Geometry: see drawing. Coordinates: mm, zero at the bounding-box minimum. Give positions to 0.01 mm unless a question says otherwise; leave off trailing zeros. Order: outer loops, then holes, each group sorted by start corner. A loop starts at its lowest first (then second) coordinate and runs counter-clockwise, first axis right, second up. Notation, with made-up numbers: (44.5, 25.5) -> (80.5, 25.5) arc R14 cw to (80.5, 52.5) -> close; hole circle Ø7 at (-28.5, -27). An arc over 180 degrees is marked (long way). One line per item, written item: value. Start each with the question number.
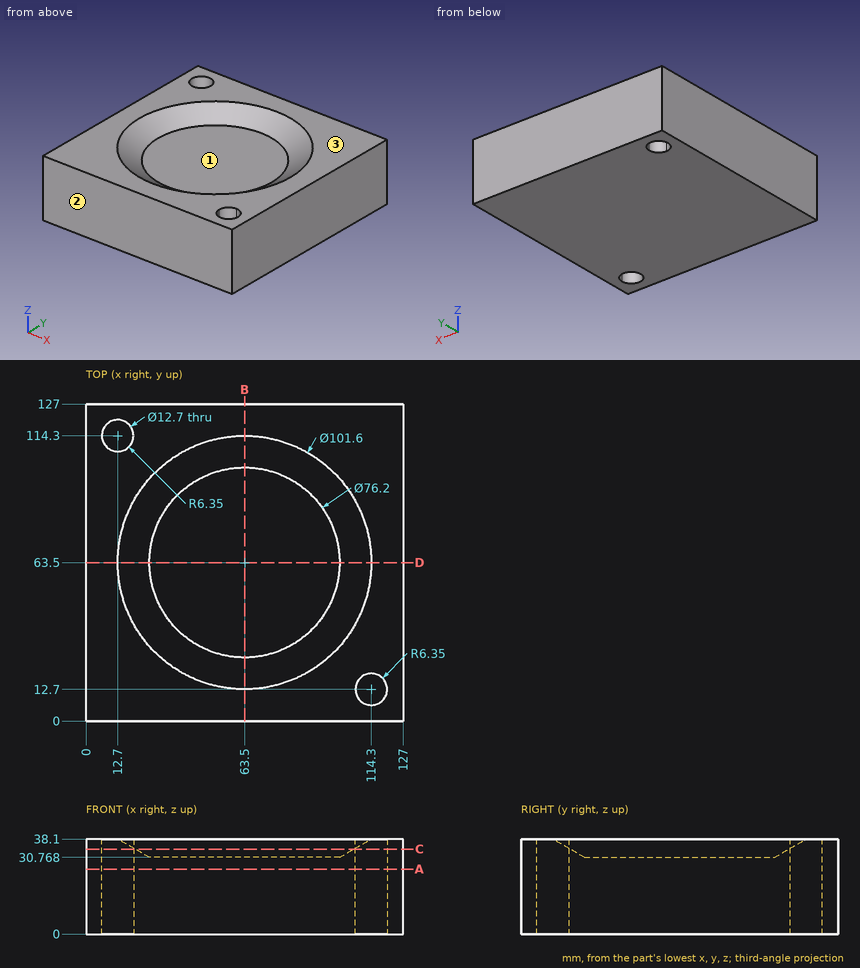
1. Cut plane B-B, the plane x = 63.5. Return loops of the section in (y, z), then the cut area to 3 significant figures.
2. Cut plane C-C, the plane z = 34. Return loops of the section in (x, y), then the cut area to 3 significant figures.
3. Pin query (flat end, axial travel): P1, Ø3, axis at x = 67.5, y = 35, coming from the +Z side; P2, Ø7.5, axis at x = 12.7, y = 114.3, coming from the -Z side. Return the tip coordinate at first contact, or that it passes through.
4. Cut plane A-A, the plane z = 26. Return loops of the section in (x, y), then the cut area to 3 significant figures.
5. Material intervals for L1, parallel to X at y = 114.3, z = 12; L2, parallel to Z at x = 43.5, y = 83; L3, parallel to Y at x = 12, z = 21, sorted ascending. Write a range as [from, to].
6. Draft query along Y for the marked faces 1, 2 and 3. Return one class per face: pulls with the +Y half, pulls with the -Y half, needs draft (parallel to the pull), parting line crosses it, or undercut.
Answers follow:
1. outline: (0, 0) -> (127, 0) -> (127, 38.1) -> (114.3, 38.1) -> (101.6, 30.77) -> (25.4, 30.77) -> (12.7, 38.1) -> (0, 38.1) -> close
1. area: 4,190 mm²
2. outline: (0, 0) -> (127, 0) -> (127, 127) -> (0, 127) -> close; hole circle Ø12.7 at (12.7, 114.3); hole circle Ø87.4 at (63.5, 63.5); hole circle Ø12.7 at (114.3, 12.7)
2. area: 9,880 mm²
3. P1: stops at z = 30.77
3. P2: passes through
4. outline: (0, 0) -> (127, 0) -> (127, 127) -> (0, 127) -> close; hole circle Ø12.7 at (12.7, 114.3); hole circle Ø12.7 at (114.3, 12.7)
4. area: 15,900 mm²
5. L1: x = [0, 6.35], [19.05, 127]
5. L2: z = [0, 30.77]
5. L3: y = [0, 107.99], [120.61, 127]
6. face 1: undercut
6. face 2: pulls with the -Y half
6. face 3: needs draft
